For this review, use the dimensioned drawing (mm, ordinates from the lowest corner) and the shaded views. A direction names the side the tool comes from. Round coordinates to 2 decimals unless told otherwise and drop trailing zeros. Loops run counter-clockwise (first coordinate to the right, second up) from the corner with the lowest first, then second, coordinate; pieces in that order, holes last. Notation, with made-up numbers: (-3.75, 25) - (22.25, 25) arc R15 cw to (22.25, 33) - close; hole circle Ø10 at (-7, 0). An arc over 180 degrees is marked (long way). Use one line per item in the form item = value. Start each with the question number.
(1) Wall thickness on probe 1 along X at (y, z) = (4.25, 17); probe 2 along X at (y, z) = (10, 45); probe 3 along X at (y, z) = (14.75, 111): over which ranges is each line inside the solid? List them lowest first. Write a range as [from, to].
(2) We need section C-C, the plane x = 62.5. Write out the cut boundary in (y, z), then the cut area to 3 significant figures.
(3) Machinability: for the marked faces 1 and 2, which of the approach directions +Z, -Z, +X, -X, +Y, -Y give a long, thin tool a straight path to every point of the face, cutting with its end or side? Answer none if there is none.
(4) The part is to be moulded in two halves that separate along Z. For the marked faces 3 and 4, say which applies: released by +Z, released by -Z, zero draft, split by the parting line, or undercut.
(5) We need section D-D, the plane x = 31.5. Write out the cut boundary in (y, z) (1 decimal).
(6) We need section B-B, the plane z = 82.5. Write out the cut boundary in (x, y), then the cut area to 3 significant figures.
(7) For pin 1 (4 mm diameter, centred on x = 49, y = 5.5, fed in from -Z); pin 2 (8 mm diameter, centred on x = 55, y = 18, fed in from +Z), all flat-tipped, find the tip position at first contact; note any pin that passes through.
(8) We need section A-A, the plane z = 55. Write out the cut boundary in (x, y).
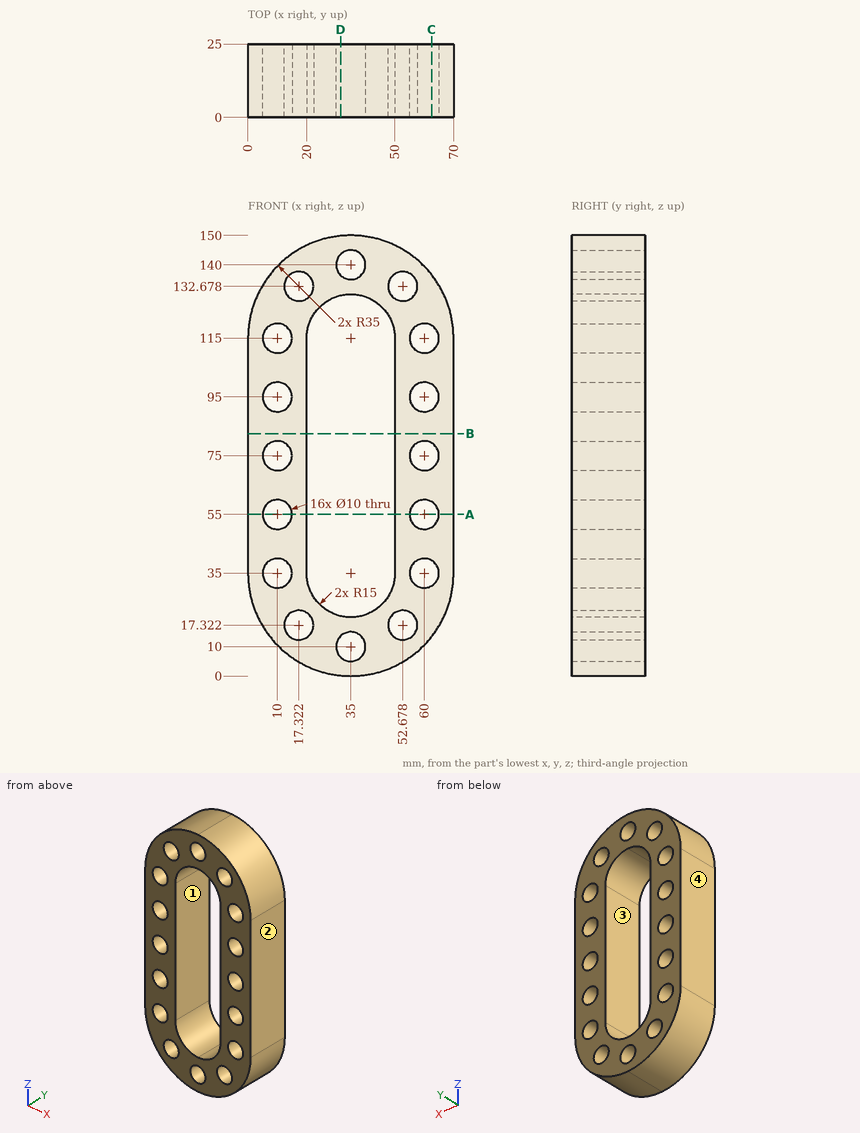
Data:
q1.probe_1 = [4.98, 12.33], [22.31, 47.69], [57.67, 65.02]
q1.probe_2 = [0, 20], [50, 70]
q1.probe_3 = [0, 7], [13, 20], [50, 57], [63, 70]
q2.outline = (0, 13.35) - (25, 13.35) - (25, 30.67) - (0, 30.67) - close; (0, 39.33) - (25, 39.33) - (25, 50.67) - (0, 50.67) - close; (0, 59.33) - (25, 59.33) - (25, 70.67) - (0, 70.67) - close; (0, 79.33) - (25, 79.33) - (25, 90.67) - (0, 90.67) - close; (0, 99.33) - (25, 99.33) - (25, 110.67) - (0, 110.67) - close; (0, 119.33) - (25, 119.33) - (25, 136.65) - (0, 136.65) - close
q2.area = 2,000 mm^2
q3.face_1 = +Y, -Y
q3.face_2 = +Z, -Z, +X, +Y, -Y
q4.face_3 = undercut
q4.face_4 = zero draft
q5.outline = (0, 0.2) - (25, 0.2) - (25, 6.4) - (0, 6.4) - close; (0, 13.6) - (25, 13.6) - (25, 20.4) - (0, 20.4) - close; (0, 129.6) - (25, 129.6) - (25, 136.4) - (0, 136.4) - close; (0, 143.6) - (25, 143.6) - (25, 149.8) - (0, 149.8) - close
q6.outline = (0, 0) - (20, 0) - (20, 25) - (0, 25) - close; (50, 0) - (70, 0) - (70, 25) - (50, 25) - close
q6.area = 1,000 mm^2
q7.pin_1 = 2.12
q7.pin_2 = 146.13
q8.outline = (0, 0) - (5, 0) - (5, 25) - (0, 25) - close; (15, 0) - (20, 0) - (20, 25) - (15, 25) - close; (50, 0) - (55, 0) - (55, 25) - (50, 25) - close; (65, 0) - (70, 0) - (70, 25) - (65, 25) - close
